Build history of the part. All positions in model axes, mm. A direction names the side the tool comes from. Coordinates: 2 decimals unless noted, no trailing zeros. Order: outer loops, then holes, each group sorted by start corner. A loop starts at its lowest first (then second) coordinate and runs counter-clockwise, first axis right, second up. Notation, with made-up numbers: (88.25, 20) - (107.25, 20) arc R23 ccw to (107.25, 32) - close; hole circle Ø2 at (-8, 16.25). An arc over 180 degrees is marked (long way). Return JSON: item names as keys, results as strings.
from build123d import *

# Parameters (mm, degrees)
F0_R     = 5.35
F0_R_2   = 3.75
F1_DEPTH = 10
F2_W     = 10.7
F2_H     = 10
F3_DEPTH = 4.75
F4_W     = 7.811706725
F4_H     = 10
F5_DEPTH = 25
F6_DEPTH = 25
F7_W     = 10.7
F7_H     = 10
F7_W_2   = 9.1
F7_H_2   = 8.4
F8_DEPTH = 0.1
F9_R     = 0.6
F10_R    = 0.75


with BuildPart() as f1:
    # F0 (on Top) → F1 (new body)
    with BuildSketch(Plane.XY):
        Circle(F0_R)
        Circle(F0_R_2, mode=Mode.SUBTRACT)
        Circle(F0_R_2)
    extrude(amount=F1_DEPTH)

    # F2 (on Right) → F3 (join)
    with BuildSketch(Plane.YZ):
        with Locations((0, 5)):
            Rectangle(F2_W, F2_H)
    extrude(amount=-F3_DEPTH)

    # F4 (on face) → F5 (cut)
    with BuildSketch(Plane(origin=(-4.75, 0, 0), x_dir=(0, -1, 0), z_dir=(-1, 0, 0))):
        with Locations((1.4441466375, 5)):
            Rectangle(F4_W, F4_H)
    extrude(amount=F5_DEPTH, mode=Mode.SUBTRACT)

    # F0 (on Top) → F6 (cut)
    with BuildSketch(Plane.XY):
        Circle(F0_R_2)
    extrude(amount=F6_DEPTH, mode=Mode.SUBTRACT)

    # F7 (on face) → F8 (join)
    with BuildSketch(Plane(origin=(-4.75, 0, 0), x_dir=(0, -1, 0), z_dir=(-1, 0, 0))):
        with Locations((0, 5)):
            Rectangle(F7_W, F7_H)
        with Locations((0, 5)):
            Rectangle(F7_W_2, F7_H_2, mode=Mode.SUBTRACT)
    extrude(amount=F8_DEPTH)

    # F9
    f9_edges = [f1.edges().sort_by_distance(p)[0] for p in [
        (-2.425, 5.35, 10),
        (-2.425, 5.35, 0),
        (-2.425, -5.35, 0),
        (-2.425, -5.35, 10),
        (-4.8, 4.55, 9.2),
        (-4.8, -4.55, 9.2),
        (-4.8, -4.55, 0.8),
        (-4.8, 4.55, 0.8),
    ]]
    fillet(f9_edges, radius=F9_R)

    # F10
    f10_edges = [f1.edges().sort_by_distance(p)[0] for p in [
        (-3.75, 0, 0),
        (-3.75, 0, 10),
    ]]
    fillet(f10_edges, radius=F10_R)


solid = f1.part
1. Cut at C-C on z = 9.75. Give the cut face in (x, y), plus the area to 3 significant figures.
Check values:
{"outline": "(-4.85, -5.24) - (0, -5.24) arc R5.24 ccw to (0, 5.24) - (-4.85, 5.24) - close; hole circle Ø7.88 at (0, 0)", "area": "45.1 mm²"}
2. Cut at B-B on y = 0. Give the cut face in (x, z), plus the area to 3 significant figures.
Check values:
{"outline": "(-4.85, 0) - (-4.5, 0) arc R0.75 ccw to (-3.75, 0.75) - (-3.75, 9.25) arc R0.75 ccw to (-4.5, 10) - (-4.85, 10) - (-4.85, 9.2) - (-4.75, 9.2) - (-4.75, 0.8) - (-4.85, 0.8) - close; (3.75, 0.75) arc R0.75 ccw to (4.5, 0) - (4.75, 0) arc R0.6 ccw to (5.35, 0.6) - (5.35, 9.4) arc R0.6 ccw to (4.75, 10) - (4.5, 10) arc R0.75 ccw to (3.75, 9.25) - close", "area": "25.5 mm²"}
3. Tool access for faces 1 (the flat face through (-4.75, 0, 5)), 2 (the flat face through (-2, 5.35, 5)): list every direction of +Z, -Z, +X, -X, +Y, -Y with a clear straight run to the whole face (end or side of a thin tool).
Check values:
{"face 1": "-X", "face 2": "+Z, -Z, +X, -X, +Y"}
4. Mould opens along X. For faces 3 (the flat face through (-2, -5.35, 5)), 4 (the flat face through (-4.85, 0.1, 0.6)), 5 (the cylindrical face through (5.35, -0.12, 4.94)), 6 (the cylindrical face through (-3.746, 0.165, 4.94)) say: pulls with the +X half, pulls with the -X half, needs draft (parallel to the pull), parting line crosses it, or undercut.
Check values:
{"face 3": "needs draft", "face 4": "pulls with the -X half", "face 5": "pulls with the +X half", "face 6": "undercut"}
5. Probe L1, parallel to Y at x = 0, z = 3.25; L2, parallel to X at y = 0, z = 4.75; L3, parallel to Y at x = 1.75, z = 1.5. List the from-to ranges inside material, lowest first.
Check values:
{"L1": "-5.35 to -3.75, 3.75 to 5.35", "L2": "-4.75 to -3.75, 3.75 to 5.35", "L3": "-5.06 to -3.32, 3.32 to 5.06"}
6. Cut at A-A on z = 8. Give the cut face in (x, y).
Check values:
{"outline": "(-4.85, -5.35) - (0, -5.35) arc R5.35 ccw to (0, 5.35) - (-4.85, 5.35) - (-4.85, 4.55) - (-4.75, 4.55) - (-4.75, -4.55) - (-4.85, -4.55) - close; hole circle Ø7.5 at (0, 0)"}
